Read the model definition and answer for the solid it produces. Units are mm, in the model's axes. Face numbers are marked on the shaded views. A direction names the side the tool comes from. Give positions to 0.01 mm unless a question says otherwise; leave off trailing zeros. Write each loop counter-clockwise with the first axis right and the second up, starting at its lowest first coordinate (ties: lowest second). Pieces come first, ordered by that corner, then holes. Notation, with made-up numbers: (71, 68.25) -> (89, 68.25) arc R9 ccw to (89, 73.25) -> close; hole circle Ø4 at (-37, 74.5). An arc over 180 degrees is marked (long way). Use a Markdown table: item, result.
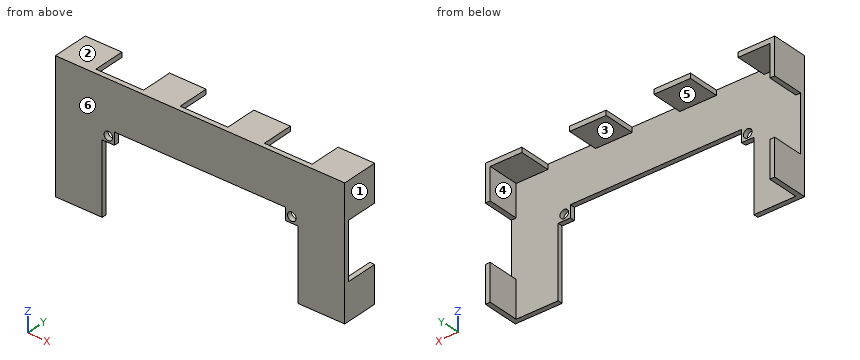
Autodesk Inventor part; units mm, degrees
ref_plane "YZ Plane" through (0, 0, 0) normal (1, 0, 0) x (0, 1, 0)
ref_plane "XZ Plane" through (0, 0, 0) normal (0, 1, 0) x (-1, 0, 0)
ref_plane "XY Plane" through (0, 0, 0) normal (0, 0, 1) x (1, 0, 0)
sketch "Sketch1" plane through (0, 0, 0) normal (0, 1, 0) x (-1, 0, 0)
  circle A0 centre (37.593, 4.5441) radius 1.75
  circle A1 centre (-37.593, 4.5441) radius 1.75
  line L0 (-35.093, 7.0441) -> (-35.093, 2.0441)
  circle A2 centre (-37.593, 4.5441) radius 1.75
  line L1 (-35.093, 7.0441) -> (35.093, 7.0441)
  line L2 (35.093, 7.0441) -> (35.093, 2.0441)
  circle A3 centre (37.593, 4.5441) radius 1.75
  line L3 (40.093, 2.0441) -> (40.093, -27.1071)
  line L4 (-40.093, -27.1071) -> (-40.093, 2.0441)
  line L5 (35.093, 2.0441) -> (40.093, 2.0441)
  line L6 (-35.093, 2.0441) -> (-40.093, 2.0441)
  line L7 (-59.2989, -27.1071) -> (-59.2989, 26)
  line L8 (-59.2989, 26) -> (59.2989, 26)
  line L9 (59.2989, 26) -> (59.2989, -27.1071)
  line L10 (59.2989, -27.1071) -> (40.093, -27.1071)
  line L11 (-40.093, -27.1071) -> (-59.2989, -27.1071)
  point P0 (0, 0)
  point P1 (0, 0)
extrude "Extrusion1" add sketch "Sketch1" along normal blind 3
sketch "Sketch3" plane through (0, 3, 0) normal (0, 1, 0) x (1, 0, 0)
  line L0 (-59.2989, -26) -> (-59.2989, -11)
  line L1 (-59.2989, 27.1071) -> (-59.2989, -26)
  line L2 (-59.2989, -26) -> (-44.2989, -26)
  line L3 (-59.2989, -26) -> (59.2989, -26)
  line L4 (-59.2989, -11) -> (-57.2989, -11)
  line L5 (-57.2989, -11) -> (-57.2989, -24)
  line L6 (-57.2989, -24) -> (-44.2989, -24)
  line L7 (-44.2989, -24) -> (-44.2989, -26)
  line L8 (0, 0) -> (0, 7) construction
  line L9 (59.2989, -26) -> (59.2989, -11)
  line L10 (59.2989, -26) -> (44.2989, -26)
  line L11 (59.2989, -11) -> (57.2989, -11)
  line L12 (57.2989, -11) -> (57.2989, -24)
  line L13 (57.2989, -24) -> (44.2989, -24)
  line L14 (44.2989, -24) -> (44.2989, -26)
  line L15 (-24.7663, -26) -> (-24.7663, -24)
  line L16 (-24.7663, -24) -> (-9.7663, -24)
  line L17 (-9.7663, -24) -> (-9.7663, -26)
  line L18 (-24.7663, -26) -> (-9.7663, -26)
  line L19 (24.7663, -26) -> (9.7663, -26)
  line L20 (9.7663, -26) -> (9.7663, -24)
  line L21 (9.7663, -24) -> (24.7663, -24)
  line L22 (24.7663, -24) -> (24.7663, -26)
  line L23 (-59.2989, 27.1071) -> (-59.2989, 12.1071)
  line L24 (-59.2989, 12.1071) -> (-57.2989, 12.1071)
  line L25 (-57.2989, 12.1071) -> (-57.2989, 27.1071)
  line L26 (-40.093, 27.1071) -> (-59.2989, 27.1071)
  line L27 (-59.2989, 27.1071) -> (-57.2989, 27.1071)
  line L28 (59.2989, 27.1071) -> (59.2989, 12.1071)
  line L29 (59.2989, 12.1071) -> (57.2989, 12.1071)
  line L30 (57.2989, 12.1071) -> (57.2989, 27.1071)
  line L31 (59.2989, 27.1071) -> (57.2989, 27.1071)
  dimension "d3" = 15
  dimension "d4" = 2
  dimension "d5" = 88.5979
  dimension "d6" = 19.5327
  dimension "d7" = 15
  dimension "d8" = 19.5327
  dimension "d9" = 15
  dimension "d10" = 2
  dimension "d11" = 15
  dimension "d12" = 2
  dimension "d15" = 2
  dimension "d16" = 2
extrude "Extrusion2" add sketch "Sketch3" along normal blind 13
sketch "Sketch5" plane through (0, 0, 0) normal (0, -1, 0) x (1, 0, 0)
  circle A0 centre (37.593, 4.5441) radius 1.75
  circle A1 centre (-37.593, 4.5441) radius 1.75
  line L0 (-59.2989, -27.1071) -> (-40.093, -27.1071)
  line L1 (-40.093, -27.1071) -> (-40.093, 2.0441)
  line L2 (-40.093, 2.0441) -> (-35.093, 2.0441)
  line L3 (-35.093, 2.0441) -> (-35.093, 7.0441)
  line L4 (-35.093, 7.0441) -> (35.093, 7.0441)
  line L5 (35.093, 7.0441) -> (35.093, 2.0441)
  line L6 (35.093, 2.0441) -> (40.093, 2.0441)
  line L7 (40.093, 2.0441) -> (40.093, -27.1071)
  line L8 (40.093, -27.1071) -> (59.2989, -27.1071)
  line L9 (59.2989, -27.1071) -> (59.2989, 26)
  line L10 (59.2989, 26) -> (-59.2989, 26)
  line L11 (-59.2989, 26) -> (-59.2989, -27.1071)
  point P0 (0, 0)
extrude "Extrusion3" cut sketch "Sketch5" against normal blind 1
properties part number "cover back i2c"
Item 1: A tool of negligible diameter and unlimited length cuts with its end or side. For the marked faces 5 and 6, from which of +Z, -Z, +X, -X, +Y, -Y can it reach the whole face along a straight path? Write none if from no direction.
Return value:
| item | result |
|---|---|
| face 5 | -Z, +Y |
| face 6 | +Z, -Z, +X, -X, -Y |
Item 2: A cutting plane is placed at B-B (y = 8). Give the vertices of the cut face in (x, z).
Return value:
| item | result |
|---|---|
| outline | (-59.3, -27.11) -> (-57.3, -27.11) -> (-57.3, -12.11) -> (-59.3, -12.11) -> close; (-59.3, 11) -> (-57.3, 11) -> (-57.3, 24) -> (-44.3, 24) -> (-44.3, 26) -> (-59.3, 26) -> close; (-24.77, 24) -> (-9.77, 24) -> (-9.77, 26) -> (-24.77, 26) -> close; (9.77, 24) -> (24.77, 24) -> (24.77, 26) -> (9.77, 26) -> close; (44.3, 24) -> (57.3, 24) -> (57.3, 11) -> (59.3, 11) -> (59.3, 26) -> (44.3, 26) -> close; (57.3, -27.11) -> (59.3, -27.11) -> (59.3, -12.11) -> (57.3, -12.11) -> close |
Item 3: Each of these flat-tipped pins is pushed along its axis until it touches: P1, Ø6.5, axis at x = 14.5, y = 9.5, coming from the -Z side; P2, Ø4.5, axis at x = -37.59, z = 4.54, coming from the +Y side; P3, Ø1, axis at x = 37, y = 2.5, coming from the -Z side; P4, Ø4, axis at x = 37.59, z = 4.54, coming from the -Y side. Where does it stop, or does it pass through?
Return value:
| item | result |
|---|---|
| P1 | z = 24 |
| P2 | y = 3 |
| P3 | z = 2.04 |
| P4 | y = 1 |
Item 4: A cutting plane is placed at C-C (z = -23). Give the vertices of the cut face in (x, y).
Return value:
| item | result |
|---|---|
| outline | (-59.3, 1) -> (-40.09, 1) -> (-40.09, 3) -> (-57.3, 3) -> (-57.3, 16) -> (-59.3, 16) -> close; (40.09, 1) -> (59.3, 1) -> (59.3, 16) -> (57.3, 16) -> (57.3, 3) -> (40.09, 3) -> close |
Item 5: A cutting plane is placed at D-D (x = -22). Give the vertices of the cut face in (y, z), then the cut area to 3 significant figures.
Return value:
| item | result |
|---|---|
| outline | (1, 7.04) -> (3, 7.04) -> (3, 24) -> (16, 24) -> (16, 26) -> (1, 26) -> close |
| area | 63.9 mm^2 |
Item 6: Straight lines are drawn through the part: line 1 along X through (y, z) = (13.5, -16.5); line 2 along X through (y, z) = (2.75, -9); line 3 along Y through (x, z) = (54, 22.5). For each, find the intervals that lie inside material, in ascending order. Write a range as [from, to].
Return value:
| item | result |
|---|---|
| line 1 | [-59.3, -57.3], [57.3, 59.3] |
| line 2 | [-59.3, -40.09], [40.09, 59.3] |
| line 3 | [1, 3] |
Item 7: A cutting plane is placed at A-A (z = -4). Give the vertices of the cut face in (x, y).
Return value:
| item | result |
|---|---|
| outline | (-59.3, 1) -> (-40.09, 1) -> (-40.09, 3) -> (-59.3, 3) -> close; (40.09, 1) -> (59.3, 1) -> (59.3, 3) -> (40.09, 3) -> close |
Item 8: For a pull along X with two mould halves and no side action, classify the marked faces 1, 2, 3 and 4 as +X half, -X half, draft (parallel to the pull), parting line (faces both ways), or undercut.
Return value:
| item | result |
|---|---|
| face 1 | +X half |
| face 2 | draft |
| face 3 | undercut |
| face 4 | undercut |
